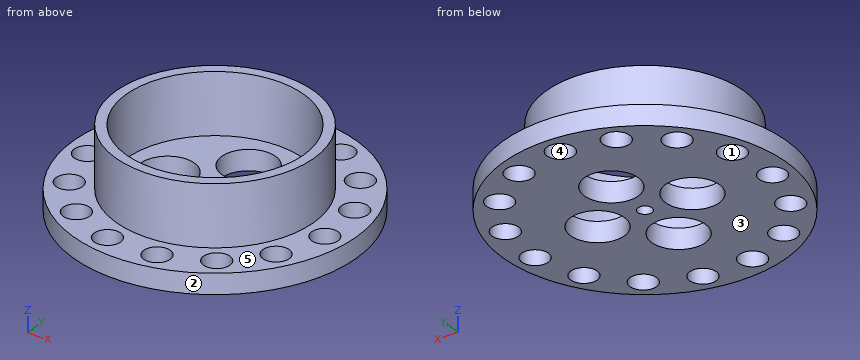
from build123d import *

# Parameters (mm, degrees)
F0_R     = 35
F0_R_2   = 3.2880949383
F0_R_3   = 24.5
F0_R_4   = 22
F0_R_5   = 6.6571375288
F0_R_6   = 1.75
F1_DEPTH = 5
F2_DEPTH = 20
F3_DEPTH = 3


with BuildPart() as f1:
    # F0 (on Top) → F1 (new body)
    with BuildSketch(Plane.XY):
        Circle(F0_R)
        with Locations((-17.5033363634, -24.0912757185)):
            Circle(F0_R_2, mode=Mode.SUBTRACT)
        with Locations((-6.1912888152, -29.1277237765)):
            Circle(F0_R_2, mode=Mode.SUBTRACT)
        with Locations((-25.7888980415, -14.8892272264)):
            Circle(F0_R_2, mode=Mode.SUBTRACT)
        with Locations((-29.6153249635, -3.1126960824)):
            Circle(F0_R_2, mode=Mode.SUBTRACT)
        with Locations((6.1912888152, -29.1277237765)):
            Circle(F0_R_2, mode=Mode.SUBTRACT)
        with Locations((17.5033363634, -24.0912757185)):
            Circle(F0_R_2, mode=Mode.SUBTRACT)
        with Locations((25.7888980415, -14.8892272264)):
            Circle(F0_R_2, mode=Mode.SUBTRACT)
        with Locations((29.6153249635, -3.1126960824)):
            Circle(F0_R_2, mode=Mode.SUBTRACT)
        with Locations((-28.3209931525, 9.2020484921)):
            Circle(F0_R_2, mode=Mode.SUBTRACT)
        with Locations((-22.1297043373, 19.9256752844)):
            Circle(F0_R_2, mode=Mode.SUBTRACT)
        with Locations((-12.1119886001, 27.2039718009)):
            Circle(F0_R_2, mode=Mode.SUBTRACT)
        Circle(F0_R_3, mode=Mode.SUBTRACT)
        with Locations((28.3209931525, 9.2020484921)):
            Circle(F0_R_2, mode=Mode.SUBTRACT)
        with Locations((0, 29.7784544528)):
            Circle(F0_R_2, mode=Mode.SUBTRACT)
        with Locations((12.1119886001, 27.2039718009)):
            Circle(F0_R_2, mode=Mode.SUBTRACT)
        with Locations((22.1297043373, 19.9256752844)):
            Circle(F0_R_2, mode=Mode.SUBTRACT)
        Circle(F0_R_3)
        Circle(F0_R_4, mode=Mode.SUBTRACT)
        Circle(F0_R_4)
        with Locations((0, -11.8328090757)):
            Circle(F0_R_5, mode=Mode.SUBTRACT)
        with Locations((-11.8328090757, 0)):
            Circle(F0_R_5, mode=Mode.SUBTRACT)
        Circle(F0_R_6, mode=Mode.SUBTRACT)
        with Locations((11.8328090757, 0)):
            Circle(F0_R_5, mode=Mode.SUBTRACT)
        with Locations((0, 11.8328090757)):
            Circle(F0_R_5, mode=Mode.SUBTRACT)
    extrude(amount=F1_DEPTH)

    # F0 (on Top) → F2 (join)
    with BuildSketch(Plane.XY):
        Circle(F0_R_3)
        Circle(F0_R_4, mode=Mode.SUBTRACT)
    extrude(amount=F2_DEPTH)

    # F0 (on Top) → F3 (join)
    with BuildSketch(Plane.XY):
        Circle(F0_R)
        with Locations((-17.5033363634, -24.0912757185)):
            Circle(F0_R_2, mode=Mode.SUBTRACT)
        with Locations((-6.1912888152, -29.1277237765)):
            Circle(F0_R_2, mode=Mode.SUBTRACT)
        with Locations((-25.7888980415, -14.8892272264)):
            Circle(F0_R_2, mode=Mode.SUBTRACT)
        with Locations((-29.6153249635, -3.1126960824)):
            Circle(F0_R_2, mode=Mode.SUBTRACT)
        with Locations((6.1912888152, -29.1277237765)):
            Circle(F0_R_2, mode=Mode.SUBTRACT)
        with Locations((17.5033363634, -24.0912757185)):
            Circle(F0_R_2, mode=Mode.SUBTRACT)
        with Locations((25.7888980415, -14.8892272264)):
            Circle(F0_R_2, mode=Mode.SUBTRACT)
        with Locations((29.6153249635, -3.1126960824)):
            Circle(F0_R_2, mode=Mode.SUBTRACT)
        with Locations((-28.3209931525, 9.2020484921)):
            Circle(F0_R_2, mode=Mode.SUBTRACT)
        with Locations((-22.1297043373, 19.9256752844)):
            Circle(F0_R_2, mode=Mode.SUBTRACT)
        with Locations((-12.1119886001, 27.2039718009)):
            Circle(F0_R_2, mode=Mode.SUBTRACT)
        Circle(F0_R_3, mode=Mode.SUBTRACT)
        with Locations((28.3209931525, 9.2020484921)):
            Circle(F0_R_2, mode=Mode.SUBTRACT)
        with Locations((0, 29.7784544528)):
            Circle(F0_R_2, mode=Mode.SUBTRACT)
        with Locations((12.1119886001, 27.2039718009)):
            Circle(F0_R_2, mode=Mode.SUBTRACT)
        with Locations((22.1297043373, 19.9256752844)):
            Circle(F0_R_2, mode=Mode.SUBTRACT)
    extrude(amount=F3_DEPTH)


solid = f1.part
Here's how the part is built. I have some questions about the finished solid (model axes, mm). Face numbers are marked on the shaded views. A direction names the side the tool comes from. Coordinates: 2 decimals unless noted, no trailing zeros. Order: outer loops, then holes, each group sorted by start corner. A loop starts at its lowest first (then second) coordinate and runs counter-clockwise, first axis right, second up. Notation, with made-up numbers: M 63,58.25 L 80,58.25 A14 ccw 80,81.25 Z; hole C 43.5,78 d4. An arc over 180 degrees is marked long. Answer as CSV lines item,"result". Start each with the question number.
1. For pin 1 (6 mm diameter, centred on x = -21, z = 4, fed in from -Y); pin 2 (1 mm diameter, centred on y = 9.5, z = 8.5, fed in from +X); pin 3 (5 mm diameter, centred on x = -21, z = 8.5, fed in from +Y), each with a flat end and sliding along its axis, tell me the tip position at first contact or that it passes through.
2. I want a section at A-A, the plane x = 0. Write out the boundary of the cut face in (y, z).
3. I want a section at D-D, the plane y = -30. Write out the boundary of the cut face in (x, z).
4. I want a section at B-B, the plane y = -16. Write out the boundary of the cut face in (x, z).
5. On a 3-axis mill with a long thin cutter (end or side, diameter ignored), from which of +Z, -Z, +X, -X, +Y, -Y can I reach the whole of each face in a straight line? I mean the marked faces 4 and 5. Say none if no direction works.
6. We'd pull the mould along Y, two halves only. Please class the marked faces 1, 2 and 3: released by +Y, released by -Y, zero draft, split by the parting line, or undercut.
7. I need wall thicknesses on line 1 (Y direction, x = 0, z = 1.4); line 2 (X direction, y = -26.5, z = 2.5); line 3 (Z direction, x = 16, y = 13). Which ranges of each line are inside material? Lowest first, please. Write a range as [from, to].
8. I want a section at C-C, the plane x = -28. Write out the boundary of the cut face in (y, z).
Recorded:
1,pin 1,"stops at y = -30.02"
1,pin 2,"stops at x = 22.79"
1,pin 3,"stops at y = 16.06"
2,outline,"M -35,0 L -18.49,0 L -18.49,5 L -22,5 L -22,20 L -24.5,20 L -24.5,5 L -35,5 Z; M -5.18,0 L -1.75,0 L -1.75,5 L -5.18,5 Z; M 1.75,0 L 5.18,0 L 5.18,5 L 1.75,5 Z; M 18.49,0 L 26.49,0 L 26.49,5 L 24.5,5 L 24.5,20 L 22,20 L 22,5 L 18.49,5 Z; M 33.07,0 L 35,0 L 35,5 L 33.07,5 Z"
3,outline,"M -18.03,0 L -9.36,0 L -9.36,5 L -18.03,5 Z; M -3.02,0 L 3.02,0 L 3.02,5 L -3.02,5 Z; M 9.36,0 L 18.03,0 L 18.03,5 L 9.36,5 Z"
4,outline,"M -31.13,0 L -28.88,0 L -28.88,5 L -31.13,5 Z; M -22.69,0 L -5.19,0 L -5.19,5 L -15.1,5 L -15.1,20 L -18.55,20 L -18.55,5 L -22.69,5 Z; M 5.19,0 L 22.69,0 L 22.69,5 L 18.55,5 L 18.55,20 L 15.1,20 L 15.1,5 L 5.19,5 Z; M 28.88,0 L 31.13,0 L 31.13,5 L 28.88,5 Z"
5,face 4,"+Z, -Z"
5,face 5,"+Z"
6,face 1,"undercut"
6,face 2,"split by the parting line"
6,face 3,"zero draft"
7,line 1,"y = [-35, -18.49], [-5.18, -1.75], [1.75, 5.18], [18.49, 26.49], [33.07, 35]"
7,line 2,"x = [-22.86, -19.74], [-15.27, -8.17], [-4.21, 4.21], [8.17, 15.27], [19.74, 22.86]"
7,line 3,"z = [0, 5]"
8,outline,"M -21,0 L -17.32,0 L -17.32,5 L -21,5 Z; M -12.46,0 L -5.98,0 L -5.98,5 L -12.46,5 Z; M -0.25,0 L 5.93,0 L 5.93,5 L -0.25,5 Z; M 12.47,0 L 21,0 L 21,5 L 12.47,5 Z"
